```python
from build123d import *

# Parameters (mm, degrees)
F0_R          = 3.5
F0_R_2        = 20
F1_DEPTH      = 3
F0_W          = 220
F0_H          = 3
F2_DEPTH      = 3
F2_DEPTH_BACK = 29
F3_R          = 5
F0_W_2        = 80
F4_DEPTH      = 3
F4_DEPTH_BACK = 22
F5_R          = 3
F6_W          = 3
F6_H          = 16
F7_DEPTH      = 80
F8_R          = 3


with BuildPart() as f1:
    # F0 (on Front) → F1 (new body)
    with BuildSketch(Plane.XZ):
        with BuildLine():
            Line((41.5, -142.5), (110, -142.5))
            Line((110, -142.5), (110, 139.5))
            Line((110, 139.5), (-110, 139.5))
            Line((-110, 139.5), (-110, -142.5))
            Line((-110, -142.5), (-41.5, -142.5))
            Line((-41.5, -142.5), (-41.5, -141.25))
            ThreePointArc((-41.5, -141.25), (-41.2803300859, -140.7196699141), (-40.75, -140.5))
            ThreePointArc((-40.75, -140.5), (-40.2196699141, -140.7196699141), (-40, -141.25))
            Line((-40, -141.25), (-40, -142.5))
            Line((-40, -142.5), (40, -142.5))
            Line((40, -142.5), (40, -141.25))
            ThreePointArc((40, -141.25), (40.2196699141, -140.7196699141), (40.75, -140.5))
            ThreePointArc((40.75, -140.5), (41.2803300859, -140.7196699141), (41.5, -141.25))
            Line((41.5, -141.25), (41.5, -142.5))
        make_face()
        with BuildLine():
            ThreePointArc((-65.5, -124.5), (-68.6819805153, -123.1819805153), (-70, -120))
            Line((-70, -120), (-70, -112))
            ThreePointArc((-70, -112), (-68.6819805153, -108.8180194847), (-65.5, -107.5))
            ThreePointArc((-65.5, -107.5), (-62.3180194847, -108.8180194847), (-61, -112))
            Line((-61, -112), (-61, -120))
            ThreePointArc((-61, -120), (-62.3180194847, -123.1819805153), (-65.5, -124.5))
        make_face(mode=Mode.SUBTRACT)
        with Locations((-28.5, -52.5)):
            Circle(F0_R, mode=Mode.SUBTRACT)
        with BuildLine():
            ThreePointArc((64.5, -107.5), (67.6819805153, -108.8180194847), (69, -112))
            Line((69, -112), (69, -120))
            ThreePointArc((69, -120), (67.6819805153, -123.1819805153), (64.5, -124.5))
            ThreePointArc((64.5, -124.5), (61.3180194847, -123.1819805153), (60, -120))
            Line((60, -120), (60, -112))
            ThreePointArc((60, -112), (61.3180194847, -108.8180194847), (64.5, -107.5))
        make_face(mode=Mode.SUBTRACT)
        with Locations((42.5, -52.5)):
            Circle(F0_R, mode=Mode.SUBTRACT)
        with BuildLine():
            ThreePointArc((-90, 56.5), (-88.5355339059, 60.0355339059), (-85, 61.5))
            Line((-85, 61.5), (-73, 61.5))
            ThreePointArc((-73, 61.5), (-69.4644660941, 60.0355339059), (-68, 56.5))
            ThreePointArc((-68, 56.5), (-69.4644660941, 52.9644660941), (-73, 51.5))
            Line((-73, 51.5), (-85, 51.5))
            ThreePointArc((-85, 51.5), (-88.5355339059, 52.9644660941), (-90, 56.5))
        make_face(mode=Mode.SUBTRACT)
        with Locations((0, 56.5)):
            Circle(F0_R_2, mode=Mode.SUBTRACT)
        with BuildLine():
            Line((73, 61.5), (85, 61.5))
            ThreePointArc((85, 61.5), (88.5355339059, 60.0355339059), (90, 56.5))
            ThreePointArc((90, 56.5), (88.5355339059, 52.9644660941), (85, 51.5))
            Line((85, 51.5), (73, 51.5))
            ThreePointArc((73, 51.5), (69.4644660941, 52.9644660941), (68, 56.5))
            ThreePointArc((68, 56.5), (69.4644660941, 60.0355339059), (73, 61.5))
        make_face(mode=Mode.SUBTRACT)
    extrude(amount=F1_DEPTH)

    # F0 (on Front) → F2 (join, two sides)
    with BuildSketch(Plane.XZ) as f2_sk:
        with Locations((0, 141)):
            Rectangle(F0_W, F0_H)
    extrude(amount=F2_DEPTH)
    extrude(f2_sk.sketch, amount=-F2_DEPTH_BACK)

    # F3
    f3_edges = [f1.edges().sort_by_distance(p)[0] for p in [
        (0, -3, 142.5),
        (0, 0, 139.5),
    ]]
    fillet(f3_edges, radius=F3_R)

    # F0 (on Front) → F4 (join, two sides)
    with BuildSketch(Plane.XZ) as f4_sk:
        with Locations((0, -144)):
            Rectangle(F0_W_2, F0_H)
    extrude(amount=F4_DEPTH)
    extrude(f4_sk.sketch, amount=-F4_DEPTH_BACK)

    # F5
    f5_edges = [f1.edges().sort_by_distance(p)[0] for p in [
        (0, -3, -145.5),
    ]]
    fillet(f5_edges, radius=F5_R)

    # F6 (on face) → F7 (join)
    with BuildSketch(Plane(origin=(-40, 0, 0), x_dir=(0, -1, 0), z_dir=(-1, 0, 0))):
        with Locations((-20.5, -134.5)):
            Rectangle(F6_W, F6_H)
    extrude(amount=-F7_DEPTH)

    # F8
    f8_edges = [f1.edges().sort_by_distance(p)[0] for p in [
        (0, 22, -145.5),
        (0, 19, -142.5),
    ]]
    fillet(f8_edges, radius=F8_R)


solid = f1.part
```
Input: part model. Units: mm. Frame: model coordinates. A direction names the side the tool comes from. Coordinates: 2 decimals unless noted, no trailing zeros. Loops run counter-clockwise (first coordinate to the right, second up) from the corner with the lowest first, then second, coordinate; pieces in that order, holes last. Notation, with made-up numbers: M -12.75,44 L 26.25,44 A20 ccw 26.25,51 Z; hole C 53,61.5 d4. An arc over 180 degrees is marked long. Use a Markdown table: item, result. Add a question column.
1) Section C-C, the plane z = -52.5. Return the cut outline in (x, y), plus the area to 3 significant figures.
2) Section A-A, the plane y = 11. Return the cut outline in (x, z).
3) Section D-D, the plane z = 68. Return the cut outline in (x, y).
4) Draft query along Z for faces 4 (the flat face through (-2, 17, 139.5)), 5 (the flat face through (-2, 15, 142.5)), 6 (the flat face through (110, -1, -1)). Return one class per face: +Z half, -Z half, draft (parallel to the pull), parting line (faces both ways), or undercut.
5) Line query: L1, parallel to Z at x = 13.5, y = 11.5; L2, parallel to Y at x = 12.5, z = 38; L3, parallel to Z at x = -45.5, y = 13. Output: solid intervals per line, ascending. Write a range as from..to.
6) Section B-B, the plane x = 0. Return the cut outline in (y, z), plus the area to 3 significant figures.
7) Set-up query: faces 1 (the flat face through (-1, 22, -135)), 2 (the cylindrical face through (-4.336, -1.479, 36.976)), 3 (the flat face through (-1, 8, -142.5)). Return all of +Z, -Z, +X, -X, +Y, -Y with unobstructed straight access to the full face (end or side cutting, diameter ignored); none if empty.
8) Pin query (flat end, axial travel): P1, Ø2.5, axis at x = 78.5, y = -1.5, coming from the -Z side; P2, Ø6.5, axis at x = -28.5, z = -52.5, coming from the -Y side; P3, Ø3, axis at x = -48.5, y = 18.5, coming from the -Z side; P4, Ø2.5, axis at x = -77.5, y = -2, coming from the +Z side. Return the tip coordinate at first contact, or that it passes through.
Answer below:
| question | item | result |
|---|---|---|
| 1 | outline | M -110,-3 L -32,-3 L -32,0 L -110,0 Z; M -25,-3 L 39,-3 L 39,0 L -25,0 Z; M 46,-3 L 110,-3 L 110,0 L 46,0 Z |
| 1 | area | 618 mm2 |
| 2 | outline | M -110,139.5 L 110,139.5 L 110,142.5 L -110,142.5 Z; M -40,-145.5 L 40,-145.5 L 40,-142.5 L -40,-142.5 Z |
| 3 | outline | M -110,-3 L -16.36,-3 L -16.36,0 L -110,0 Z; M 16.36,-3 L 110,-3 L 110,0 L 16.36,0 Z |
| 4 | face 4 | undercut |
| 4 | face 5 | +Z half |
| 4 | face 6 | draft |
| 5 | L1 | -145.5..-142.5, 139.5..142.5 |
| 5 | L2 | -3..0 |
| 5 | L3 | 139.5..142.5 |
| 6 | outline | M -3,-142.5 A3 ccw 0,-145.5 L 19,-145.5 A3 ccw 22,-142.5 L 22,-126.5 L 19,-126.5 L 19,-139.5 A3 cw 16,-142.5 L 0,-142.5 L 0,36.5 L -3,36.5 Z; M -3,76.5 L 0,76.5 L 0,134.5 A5 cw 5,139.5 L 29,139.5 L 29,142.5 L 2,142.5 A5 ccw -3,137.5 Z |
| 6 | area | 943 mm2 |
| 7 | face 1 | -Z, +X, -X, +Y |
| 7 | face 2 | +Y, -Y |
| 7 | face 3 | +X, -X |
| 8 | P1 | z = -142.5 |
| 8 | P2 | through |
| 8 | P3 | z = 139.5 |
| 8 | P4 | z = 141.68 |
